from build123d import *

# Parameters (mm, degrees)
BOSS_EXTRUDE1_DEPTH = 0.635
CIRPATTERN1_COUNT   = 4


with BuildPart() as part:
    # Sketch1 → Revolve1 (revolve)
    with BuildSketch(Plane.XY):
        Polygon((-30.401242848, 69.85), (-1.650713674, 69.85), (36.187462891, 38.1), (37.003803155, 39.072876443), (-1.188471476, 71.12), (-30.401242848, 71.12), align=None)
    revolve(axis=Axis((0, 0, 0), (-1, 0, 0)))



with BuildPart() as body_2:
    # Sketch2 → Revolve2 (revolve)
    with BuildSketch(Plane.XY):
        Polygon((0.784405442, 49.827123557), (1.600745706, 50.8), (59.468872152, 2.242876443), (58.652531887, 1.27), align=None)
    revolve(axis=Axis((0, 0, 0), (-1, 0, 0)))


with BuildPart() as part_1:
    add(part.part)

    add(body_2.part)  # Boss-Extrude1 merges body 2
    # Sketch3 → Boss-Extrude1 (add, symmetric)
    with BuildSketch(Plane.XY):
        Polygon((30.952144014, 42.599035585), (36.107835241, 38.272896978), (27.427825795, 27.928464538), (22.272134568, 32.254603145), align=None)
    boss_extrude1 = extrude(amount=BOSS_EXTRUDE1_DEPTH, both=True)

    # CirPattern1: Boss-Extrude1 ×4 about axis
    cirpattern1_axis = Axis((0, 0, 0), (1, 0, 0))
    for i in range(1, CIRPATTERN1_COUNT):
        add(boss_extrude1.rotate(cirpattern1_axis, i * 360 / CIRPATTERN1_COUNT))


solid = part_1.part
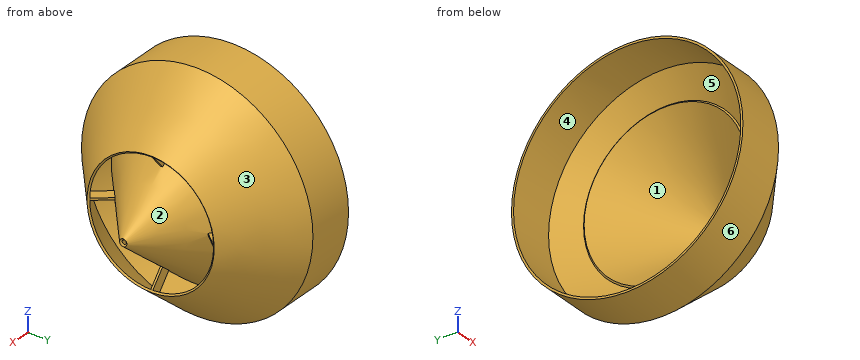
Input: part model. Units: mm. Frame: model coordinates. Face numbers are marked on the shaded views. A direction names the side the tool comes from. Coordinates: 2 decimals unless noted, no trailing zeros. Loops run counter-clockwise (first coordinate to the right, second up) from the corner with the lowest first, then second, coordinate; pieces in that order, holes last. Notation, with made-up numbers: (13.25, 18) - (65.25, 18) arc R11 cw to (65.25, 24) - close; hole circle Ø3 at (53, -1). An arc over 180 degrees is marked (long way). Answer in a Markdown table with one row per item. Add a question column.
Item 1: Mould query, pull axis Y, two halves, no side actions, for the marked faces 1, 2 and 3. Classes: released by +Y, released by -Y, zero draft, split by the parting line, or undercut.
Item 2: Section query A-A on x = -22. Return the cut outline in (y, z).
Item 3: Contact query for flat-ended pins moving along their axis: P1, Ø5, axis at y = 0, z = 55.5, coming from the -X side; P2, Ø6.5, axis at x = 29, y = 37, coming from the -Z side; P3, Ø6.5, axis at x = 30, y = -38.5, coming from the -Z side. Output: stop coordinate, or through.
Item 4: Section query B-B on y = -5.5. State how many separate pieces and enclosed holes the cut face has, then the cut area to 3 significant figures.
Item 5: Access query for the marked faces 4, 5 and 6. Directions: +Z, -Z, +X, -X, +Y, -Y. A direction counts if a zero-diameter tool reaches every point of the face in a straight line with its end or side. Return the directions, or none.
Item 6: Line query: line 1 along Y through (x, z) = (-24, 0); line 2 along Y through (x, z) = (22, 15). Output: solid intervals per line, ascending. Write a range as [from, to].
Recorded:
| question | item | result |
|---|---|---|
| 1 | face 1 | undercut |
| 1 | face 2 | undercut |
| 1 | face 3 | split by the parting line |
| 2 | outline | circle Ø142.24 at (0, 0); hole circle Ø139.7 at (0, 0) |
| 3 | P1 | x = 12.47 |
| 3 | P2 | z = -32.77 |
| 3 | P3 | z = -29.79 |
| 4 | separate pieces | 3 |
| 4 | enclosed holes | 0 |
| 4 | area | 398 mm^2 |
| 5 | face 4 | -X |
| 5 | face 5 | none |
| 5 | face 6 | +X, -X |
| 6 | line 1 | [-71.12, -69.85], [69.85, 71.12] |
| 6 | line 2 | [-49.44, -47.7], [-30.16, -28.3], [28.3, 30.16], [47.7, 49.44] |
